Read the model definition and answer for the solid it produces. Units are mm, in the model's axes. Face numbers are marked on the shaded views. A direction names the side the tool comes from. Give positions to 0.01 mm unless a question says otherwise; leave off trailing zeros. Loops run counter-clockwise (first coordinate to the right, second up) from the corner with the lowest first, then second, coordinate; pieces in that order, holes last. Notation, with made-up numbers: (79.25, 59) - (101.25, 59) arc R21 ccw to (101.25, 86) - close; hole circle Ø7 at (62, 47.25). An arc over 180 degrees is marked (long way). Put each result on its own line as item: value. Start each with the question number.
1. For the marked faces 5, 6 and 7, determine the directions among +Z, -Z, +X, -X, +Y, -Y from which every point of the face is accessible in a straight line to the end or side of a thin tool.
2. A cutting plane is placed at D-D, the plane y = -92.5. Determine the outline of the cut face in (x, z), plus the area to 3 significant figures.
3. A cutting plane is placed at C-C, the plane y = -134. Determine the outline of the cut face in (x, z), plus the area to 3 significant figures.
4. Given pin 1 Ø10.5 at (x, z) = (10, 20) entering from -Y; pin 2 Ø4 at (y, z) = (-45, 24.5) entering from +X; pin 3 Ø13.5 at (y, z) = (-134, 20) entering from -X, each flat-ended and moving along its own axis, determine where each tip first touches the part or whether it passes through.
5. A cutting plane is placed at A-A, the plane x = 10. Determine the outline of the cut face in (y, z), plus the area to 3 significant figures.
6. For a pull along X with two mould halves and no side action, classify the marked faces 1, 2, 3 and 4 as released by +X, released by -X, zero draft, split by the parting line, or undercut.
7. A cutting plane is placed at B-B, the plane z = 20. Determine the outline of the cut face in (x, y).
8. Consider L1, parallel to X at y = -36, z = 33.5; L2, parallel to Z at x = 143, y = -1; L3, parallel to Z at x = 121.05, y = -134. Determine where each line is inside the solid, lowest interval first. Write a range as from..to.
```python
from build123d import *

# Parameters (mm, degrees)
F0_W     = 153
F0_H     = 40
F1_DEPTH = 4
F2_W     = 4
F2_H     = 40
F3_DEPTH = 150
F4_R     = 4.5
F5_DEPTH = 25
F6_R     = 5.15
F7_DEPTH = 123.001


with BuildPart() as f1:
    # F0 (on Front) → F1 (new body)
    with BuildSketch(Plane.XZ):
        with Locations((76.5, 20)):
            Rectangle(F0_W, F0_H)
    extrude(amount=F1_DEPTH)

    # F2 (on face) → F3 (join)
    with BuildSketch(Plane.XZ.offset(4)):
        with Locations((32, 20)):
            Rectangle(F2_W, F2_H)
        with Locations((121, 20)):
            Rectangle(F2_W, F2_H)
    extrude(amount=F3_DEPTH)

    # F4 (on face) → F5 (cut)
    with BuildSketch(Plane.XZ.offset(4)):
        with Locations((143, 20)):
            Circle(F4_R)
        with Locations((10, 20)):
            Circle(F4_R)
    extrude(amount=-F5_DEPTH, mode=Mode.SUBTRACT)

    # F6 (on face) → F7 (cut, through all)
    with BuildSketch(Plane.YZ.offset(123)):
        with Locations((-134, 20)):
            Circle(F6_R)
    extrude(amount=-F7_DEPTH, mode=Mode.SUBTRACT)


solid = f1.part
```
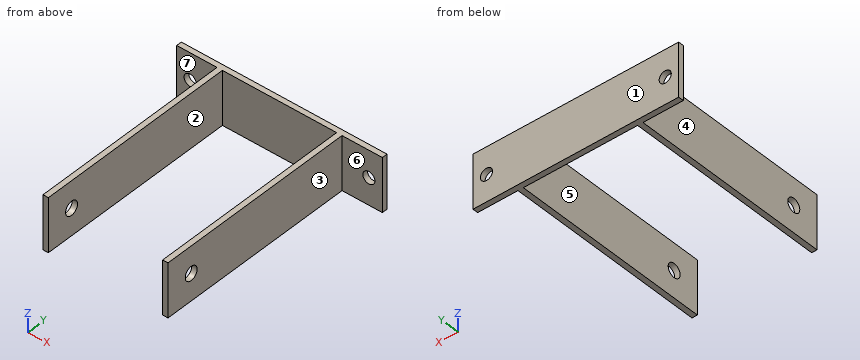
Return value:
1. face 5: +Z, -Z, -Y
1. face 6: +Z, -Z, +X, -Y
1. face 7: +Z, -Z, -X, -Y
2. outline: (30, 0) - (34, 0) - (34, 40) - (30, 40) - close; (119, 0) - (123, 0) - (123, 40) - (119, 40) - close
2. area: 320 mm2
3. outline: (30, 0) - (34, 0) - (34, 14.85) - (30, 14.85) - close; (30, 25.15) - (34, 25.15) - (34, 40) - (30, 40) - close; (119, 0) - (123, 0) - (123, 14.85) - (119, 14.85) - close; (119, 25.15) - (123, 25.15) - (123, 40) - (119, 40) - close
3. area: 238 mm2
4. pin 1: stops at y = -4
4. pin 2: stops at x = 123
4. pin 3: stops at x = 30
5. outline: (-4, 0) - (0, 0) - (0, 15.5) - (-4, 15.5) - close; (-4, 24.5) - (0, 24.5) - (0, 40) - (-4, 40) - close
5. area: 124 mm2
6. face 1: zero draft
6. face 2: undercut
6. face 3: released by +X
6. face 4: released by -X
7. outline: (0, -4) - (5.5, -4) - (5.5, 0) - (0, 0) - close; (14.5, -4) - (30, -4) - (30, -128.85) - (34, -128.85) - (34, -4) - (119, -4) - (119, -128.85) - (123, -128.85) - (123, -4) - (138.5, -4) - (138.5, 0) - (14.5, 0) - close; (30, -154) - (34, -154) - (34, -139.15) - (30, -139.15) - close; (119, -154) - (123, -154) - (123, -139.15) - (119, -139.15) - close; (147.5, -4) - (153, -4) - (153, 0) - (147.5, 0) - close
8. L1: x = 30..34, 119..123
8. L2: z = 0..15.5, 24.5..40
8. L3: z = 0..14.85, 25.15..40
